Input: part model. Units: mm. Frame: model coordinates. Face numbers are marked on the shaded views. A direction names the side the tool comes from. Round coordinates to 2 decimals unless told otherwise and drop trailing zeros. Write each loop counter-clockwise with the first axis right and the second up, starting at its lowest first coordinate (ties: lowest second). Pieces come first, ordered by that corner, then holes. Notation, with made-up numbers: (-31.75, 22.5) -> (-7.75, 22.5) arc R20 ccw to (-7.75, 58.5) -> close; hole circle Ø7 at (43.5, 73). An arc over 180 degrees is marked (long way). Use CSV: the item, a comma, the result in double quotes.
Autodesk Inventor part; units mm, degrees
ref_plane "YZ Plane" through (0, 0, 0) normal (1, 0, 0) x (0, 1, 0)
ref_plane "XZ Plane" through (0, 0, 0) normal (0, 1, 0) x (-1, 0, 0)
ref_plane "XY Plane" through (0, 0, 0) normal (0, 0, 1) x (1, 0, 0)
sketch "Sketch4" plane through (0, 0, 0) normal (1, 0, 0) x (0, 1, 0)
  line L0 (0, 0) -> (-152.4, 0)
  line L1 (-152.4, 0) -> (-152.4, -133.35)
  line L2 (-152.4, -133.35) -> (0, -133.35)
  line L3 (0, -133.35) -> (0, 0)
  dimension "d10" = 152.4
  dimension "d11" = 133.35
extrude "Extrusion2" add sketch "Sketch4" along normal blind 5.08
sketch "Sketch5" plane through (5.08, 0, 0) normal (1, 0, 0) x (0, 0, -1)
  line L0 (133.35, 0) -> (0, 0)
  line L1 (66.675, 0) -> (66.675, -152.4)
  line L2 (0, -152.4) -> (133.35, -152.4)
  circle A0 centre (126.5334, -28.194) radius 1.651
  circle A1 centre (74.9714, -28.194) radius 1.651
  circle A2 centre (61.2554, -28.194) radius 1.651
  circle A3 centre (9.6934, -28.194) radius 1.651
  circle A4 centre (126.5334, -63.754) radius 1.651
  circle A5 centre (74.9714, -63.754) radius 1.651
  circle A6 centre (61.2554, -63.754) radius 1.651
  circle A7 centre (9.6934, -63.754) radius 1.651
  circle A8 centre (113.5794, -45.974) radius 2.413
  circle A9 centre (87.9254, -45.974) radius 2.413
  circle A10 centre (48.3014, -45.974) radius 2.413
  circle A11 centre (22.6474, -45.974) radius 2.413
  line L3 (66.675, 0) -> (66.675, -28.194)
  line L4 (66.675, -28.194) -> (73.533, -28.194)
  line L5 (73.533, -28.194) -> (66.675, -28.194)
  line L6 (66.675, -28.194) -> (59.817, -28.194)
  dimension "d14" = 28.194
  dimension "d15" = 6.858
  dimension "d16" = 6.858
extrude "Extrusion3" cut sketch "Sketch5" against normal blind 5.08
sketch "Sketch6" plane through (5.08, 0, 0) normal (1, 0, 0) x (0, 0, -1)
  circle A0 centre (22.6474, -45.974) radius 2.413
  circle A1 centre (48.3014, -45.974) radius 2.413
  line L0 (0, -152.4) -> (133.35, -152.4)
  circle A2 centre (35.4744, -134.874) radius 6.35
  circle A3 centre (87.9254, -45.974) radius 2.413
  circle A4 centre (113.5794, -45.974) radius 2.413
  circle A5 centre (100.7524, -134.874) radius 6.35
  point P0 (0, 0)
  dimension "d20" = 12.7
  dimension "d22" = 12.7
extrude "Extrusion4" cut sketch "Sketch6" against normal blind 5.08 contours A2 | A5
sketch "Sketch7" plane through (0, 0, 0) normal (-1, 0, 0) x (0, 0, 1)
  line L0 (-133.35, 0) -> (0, 0)
  line L1 (-66.675, 0) -> (-66.675, -152.4)
  line L2 (0, -152.4) -> (-133.35, -152.4)
  line L3 (-79.375, -107.9503) -> (-53.975, -107.9503)
  line L4 (-53.975, -107.9503) -> (-53.975, -152.4)
  line L5 (-53.975, -152.4) -> (-79.375, -152.4)
  line L6 (-79.375, -152.4) -> (-79.375, -107.9503)
  line L7 (-79.375, -107.9503) -> (-53.975, -152.4) construction
  line L8 (-53.975, -107.9503) -> (-79.375, -152.4) construction
  point P0 (-66.675, -130.1752)
  dimension "d29" = 25.4
extrude "Extrusion5" add sketch "Sketch7" along normal blind 25.4
sketch "Sketch8" plane through (0, -152.4, -79.375) normal (0, 0, -1) x (-1, 0, 0)
  line L0 (25.4, 0) -> (25.4, 44.4497)
  line L1 (0, 44.4497) -> (25.4, 44.4497)
  line L2 (25.4, 0) -> (0, 44.4497)
  point P0 (0, 152.4)
extrude "Extrusion6" cut sketch "Sketch8" against normal blind 25.4
sketch "Sketch9" plane through (5.08, 0, 0) normal (1, 0, 0) x (0, 0, -1)
  point P0 (0, 0)
properties part number "HalfBackWall"
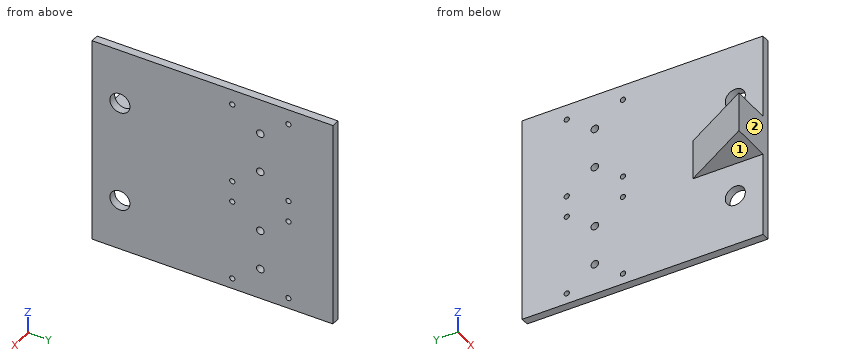
Item 1: Section query C-C on x = -20. Return the cut outline in (y, z) (3 decimals), plus the area to 3 significant figures.
Worked answers:
outline,"(-152.4, -79.375) -> (-142.95, -79.375) -> (-142.95, -53.975) -> (-152.4, -53.975) -> close"
area,"240 mm²"
Item 2: Section query B-B on y = -110.5. Return the cut outline in (x, z) (3 decimals).
Worked answers:
outline,"(-1.457, -79.375) -> (0, -79.375) -> (0, -133.35) -> (5.08, -133.35) -> (5.08, 0) -> (0, 0) -> (0, -53.975) -> (-1.457, -53.975) -> close"
Item 3: Section query A-A on z = -113. Return the cut outline in (x, y), plus the area to 3 significant figures.
Worked answers:
outline,"(0, -152.4) -> (5.08, -152.4) -> (5.08, -48.32) -> (0, -48.32) -> close; (0, -43.63) -> (5.08, -43.63) -> (5.08, 0) -> (0, 0) -> close"
area,"750 mm²"
Item 4: Line query: line 1 (X direction, y = -8.5, z = -97); line 2 (Z direction, x = -2.5, y = -131.5) (3 decimals); line 3 (Y direction, x = 4, z = -95.5). Output: solid intervals per line, ascending.
Worked answers:
line 1,"x = 0 to 5.08"
line 2,"z = -79.375 to -53.975"
line 3,"y = -152.4 to -138.44, -131.31 to 0"
Item 5: Section query D-D on z = -13. Return the cut outline in (x, y).
Worked answers:
outline,"(0, -152.4) -> (5.08, -152.4) -> (5.08, 0) -> (0, 0) -> close"
Item 6: Set-up query: the marked faces 1 and 2. Return all of +Z, -Z, +X, -X, +Y, -Y with unobstructed straight access to the full face (end or side cutting, diameter ignored); none if empty.
Worked answers:
face 1,"-Z, -X, +Y, -Y"
face 2,"+Z, -Z, +X, -X, -Y"
Item 7: First-contact query: pin 1 Ø2 at (y, z) = (-28.19, -74.97) entering from +X (3 decimals); pin 2 Ø5 at (y, z) = (-109.5, -17.5) entering from -X; pin 3 Ø5.5 at (y, z) = (-28.19, -9.69) entering from +X; pin 4 Ø3 at (x, y) = (-2, -117.5) entering from +Z (3 decimals). Flat tips, straight axial feed; report the tip coordinate or a pass-through.
Worked answers:
pin 1,"passes through"
pin 2,"stops at x = 0"
pin 3,"stops at x = 5.08"
pin 4,"stops at z = -53.975"
